Build history of the part. All positions in model axes, mm. Face numbers are marked on the shaded views. A direction names the side the tool comes from. Round coordinates to 2 decimals unless told otherwise and drop trailing zeros. Loops run counter-clockwise (first coordinate to the right, second up) from the corner with the lowest first, then second, coordinate; pieces in that order, holes last. Notation, with made-up numbers: (-39.75, -7) -> (-23.75, -7) arc R19 cw to (-23.75, 15) -> close; hole circle Ø8 at (-30, 16.5). An arc over 180 degrees is marked (long way). Put each result on its own line as item: value. Start each with the question number.
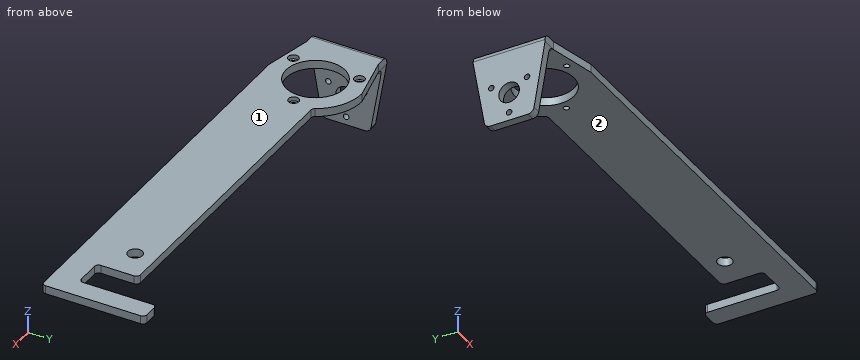
Autodesk Inventor part; units mm, degrees
ref_plane "YZ Plane" through (0, 0, 0) normal (1, 0, 0) x (0, 1, 0)
ref_plane "XZ Plane" through (0, 0, 0) normal (0, 1, 0) x (-1, 0, 0)
ref_plane "XY Plane" through (0, 0, 0) normal (0, 0, 1) x (1, 0, 0)
sketch "スケッチ1" plane through (0, 0, 0) normal (1, 0, 0) x (0, 1, 0)
  circle A0 centre (0, 0) radius 10
  circle A1 centre (0, -10) radius 1.35
  circle A2 centre (8.6603, 5) radius 1.35
  circle A3 centre (-8.6603, 5) radius 1.35
  circle A4 centre (0, 0) radius 5
  line L0 (0, 0) -> (0, 50)
  circle A5 centre (0, 50) radius 22.5
  circle A6 centre (0, 0) radius 14
  line L1 (-14, 0) -> (-22.5, 50)
  line L2 (14, 0) -> (22.5, 50)
  line L3 (0, -14) -> (-11.62, -14)
  line L4 (-11.62, -14) -> (-14, 0)
  line L5 (0, -14) -> (11.62, -14)
  line L6 (11.62, -14) -> (14, 0)
  line L7 (0, 20) -> (-17.4, 20)
  line L8 (0, 20) -> (17.4, 20)
  dimension "d0" = 20
  dimension "d1" = 2.7
  dimension "d4" = 360
  dimension "d6" = 10
  dimension "d7" = 50
  dimension "d8" = 45
  dimension "d9" = 28
extrude "押し出し1" add sketch "スケッチ1" along normal blind 4 contours A0 A1 A3 A2 | A6 L6 L4 | A6 L1 L7 L0 | L0 L8 L2 A6 | L6 L5 A6 | A6 L3 L4
sketch "スケッチ2" plane through (0, -17.4, 20) normal (0, 0, 1) x (1, 0, 0)
  line L0 (0, 17.4) -> (30, 17.4)
  circle A0 centre (30, 17.4) radius 22.5
  circle A1 centre (30, 17.4) radius 18.5
  circle A2 centre (30, 17.4) radius 14.25
  circle A3 centre (48.5, 17.4) radius 1.35
  circle A4 centre (20.75, 33.4215) radius 1.35
  circle A5 centre (20.75, 1.3785) radius 1.35
  line L1 (0, 29.02) -> (0, 34.8)
  line L2 (0, 0) -> (0, 5.78)
  line L3 (0, 34.8) -> (0, 0)
  line L4 (4, 29.02) -> (4, 34.8)
  line L5 (4, 34.8) -> (7, 34.8)
  line L6 (7, 34.8) -> (30, 39.9)
  line L7 (4, 0) -> (4, 5.78)
  line L8 (4, 0) -> (7, 0)
  line L9 (7, 0) -> (30, -5.1)
  line L10 (4, 0) -> (0, 0)
  line L11 (0, 34.8) -> (4, 34.8)
  line L12 (0, 0) -> (0, 34.8)
  line L13 (0, 34.8) -> (4, 34.8)
  dimension "d14" = 37
  dimension "d12" = 30
  dimension "d13" = 45
  dimension "d15" = 28.5
  dimension "d16" = 2.7
  dimension "d19" = 360
  dimension "d21" = 3
  dimension "d22" = 3
extrude "押し出し2" add sketch "スケッチ2" along normal blind 4 contours L3 L1 L11 L5 L6 A0 L0 | L0 A0 L9 L8 L10 L2 L3 | A1 A4 A3 A5 | A0 L6 L9
fillet "フィレット1" radius 3 2 edges at (4, 0, 20) (0, 0, 24)
fillet "フィレット2" radius 3 2 edges at (2, -11.62, -14) (2, 11.62, -14)
sketch "スケッチ7" plane through (0, -17.4, 24) normal (0, 0, 1) x (1, 0, 0)
  circle A0 centre (30, 17.4) radius 14.25
  line L0 (30, 17.4) -> (182.95, 17.4)
  line L1 (30, 17.4) -> (182.95, 17.4) construction
  circle A1 centre (182.95, 17.4) radius 3.5
  circle A2 centre (182.95, 17.4) radius 10
  line L2 (182.95, 27.4) -> (50.1556, 27.4)
  arc A3 (30, -5.1) -> (30, 39.9) centre (30, 17.4) ccw
  line L3 (182.95, 27.4) -> (315.7444, 27.4) construction
  line L4 (182.95, 7.4) -> (50.1556, 7.4)
  point P0 (0, 17.4)
  dimension "d55" = 152.95
  dimension "d56" = 0
  dimension "d57" = 7
  dimension "d58" = 20
  dimension "d59" = 180
extrude "押し出し7" add sketch "スケッチ7" against normal blind 4 contours A3 L2 A2 L0 | L0 A2 L4 A3 | A2
sketch "スケッチ8" plane through (0, -17.4, 24) normal (0, 0, 1) x (1, 0, 0)
  circle A0 centre (20.75, 33.4215) radius 1.35
  circle A1 centre (20.75, 33.4215) radius 2.5
  circle A2 centre (48.5, 17.4) radius 1.35
  circle A3 centre (48.5, 17.4) radius 2.5
  circle A4 centre (20.75, 1.3785) radius 1.35
  circle A5 centre (20.75, 1.3785) radius 2.5
  point P0 (0, 17.4)
  dimension "d63" = 5
  dimension "d64" = 5
  dimension "d65" = 5
extrude "押し出し8" cut sketch "スケッチ8" against normal blind 2 contours A0 | A1 | A3 | A4 | A5
sketch "スケッチ9" plane through (0, -17.4, 24) normal (0, 0, 1) x (1, 0, 0)
  line L0 (50.1556, 27.4) -> (182.95, 27.4)
  line L1 (182.95, 27.4) -> (197.95, 27.4)
  line L2 (7, 0) -> (30, -5.1)
  line L3 (30, -5.1) -> (197.95, -5.1)
  line L4 (197.95, -5.1) -> (197.95, 27.4)
  line L5 (197.95, -5.1) -> (222.95, -5.1)
  line L6 (222.95, -5.1) -> (222.95, 44.9)
  line L7 (222.95, 44.9) -> (212.95, 44.9)
  line L8 (197.95, 7.4) -> (212.95, 7.4)
  line L9 (212.95, 7.4) -> (212.95, 44.9)
  circle A0 centre (182.95, 17.4) radius 3.5
  circle A1 centre (182.95, 17.4) radius 10
  circle A2 centre (30, 17.4) radius 14.25
  circle A3 centre (30, 17.4) radius 22.5
  line L10 (182.95, 7.4) -> (50.1556, 7.4)
  line L11 (50.1556, 7.4) -> (182.95, 7.4)
  point P0 (0, 17.4)
  point P1 (192.95, 17.4)
  point P2 (20.4894, -2.9911)
  dimension "d68" = 15
  dimension "d69" = 25
  dimension "d70" = 50
  dimension "d71" = 10
extrude "押し出し9" add sketch "スケッチ9" against normal blind 4 contours L0 A1 L10 A3 | L1 L4 L3 A3 L10 A1 | L8 L9 L7 L6 L5 L4
fillet "フィレット4" radius 2 7 edges at (197.95, 10, 22) (50.1556, 10, 22) (212.95, 27.5, 22) (212.95, -10, 22) (222.95, 27.5, 22) (197.95, -10, 22) (222.95, -22.5, 22)
properties part number "motor_holder_2" material "アルミニウム 6061"
Item 1: Wall check: line 1 (Y direction, x = 30, z = 21); line 2 (X direction, y = -14.5, z = 6); line 3 (Y direction, x = 48, z = 23). Give the ranges that are in metal, low to high. Write a range as from..to.
Item 2: Cut at A-A on z = 0. Write the cut outline in (x, y), then the cut area to 3 significant figures.
Item 3: Drop flat-ended pins along their axis: pin 1 (10 mm diameter, centred on x = 107, y = -14, fed in from -Z); pin 2 (6 mm diameter, centred on y = 2, z = 1.5, fed in from +X); pin 3 (3 mm diameter, centred on x = 4, z = 23, fed in from -Y). Give the stop position or say it passes through.
Item 4: Cut at B-B on x = 92.5. Write the cut outline in (y, z), then the cut area to 3 significant figures.
Item 5: 3-axis set-ups, long thin cutter, end or side, ignore diameter. For the marked faces 1 and 2: which of +Z, -Z, +X, -X, +Y, -Y reach the whole face in a straight line?
Ans:
1. line 1: y = -22.5..-14.25, 14.25..22.5
1. line 2: x = 0..4
1. line 3: y = -22.5..-2.45, 2.45..13.5
2. outline: (0, -14) -> (4, -14) -> (4, -5) -> (0, -5) -> close; (0, 5) -> (4, 5) -> (4, 14) -> (0, 14) -> close
2. area: 72.0 mm2
3. pin 1: stops at z = 20
3. pin 2: stops at x = 4
3. pin 3: stops at y = -17.4
4. outline: (-22.5, 20) -> (10, 20) -> (10, 24) -> (-22.5, 24) -> close
4. area: 130 mm2
5. face 1: +Z, +X, -X, +Y, -Y
5. face 2: -Z, +X, +Y, -Y
